Read the model definition and answer for the solid it produces. Units are mm, in the model's axes. A direction names the side the tool comes from. Coordinates: 2 decimals unless noted, no trailing zeros. Loops run counter-clockwise (first coordinate to the right, second up) from the corner with the lowest first, then second, coordinate; pieces in that order, holes last. Notation, with made-up numbers: (-20.75, 49) - (3.25, 49) arc R29 ccw to (3.25, 77) - close; hole circle Ø3 at (-30, -3). An arc over 180 degrees is marked (long way). One line per question, with ' | ' between items. Start each with the question number.
Autodesk Inventor part; units mm, degrees
ref_plane "YZ Plane" through (0, 0, 0) normal (1, 0, 0) x (0, 1, 0)
ref_plane "XZ Plane" through (0, 0, 0) normal (0, 1, 0) x (-1, 0, 0)
ref_plane "XY Plane" through (0, 0, 0) normal (0, 0, 1) x (1, 0, 0)
sketch "Sketch1" plane through (0, 0, 0) normal (0, 1, 0) x (-1, 0, 0)
  line L0 (0, 0) -> (57, 0)
  line L1 (57, 0) -> (57, -77)
  line L2 (57, -77) -> (0, -77)
  line L3 (0, -77) -> (0, 0)
  line L4 (53.5, -3.5) -> (3.5, -3.5) construction
  line L5 (3.5, -3.5) -> (3.5, -73.5) construction
  line L6 (3.5, -73.5) -> (53.5, -73.5) construction
  line L7 (53.5, -73.5) -> (53.5, -3.5) construction
  line L8 (52, -5) -> (5, -5)
  line L9 (5, -5) -> (5, -72)
  line L10 (5, -72) -> (52, -72)
  line L11 (52, -72) -> (52, -5)
  circle A0 centre (53.5, -3.5) radius 1.8
  circle A1 centre (53.5, -73.5) radius 1.8
  circle A2 centre (3.5, -3.5) radius 1.8
  circle A3 centre (3.5, -73.5) radius 1.8
  dimension "d0" = 57
  dimension "d1" = 77
  dimension "d2" = 50
  dimension "d3" = 70
  dimension "d4" = 3.5
  dimension "d5" = 3.5
  dimension "d6" = 67
  dimension "d7" = 47
  dimension "d8" = 1.5
  dimension "d9" = 1.5
  dimension "d10" = 3.6
  dimension "d11" = 3.6
  dimension "d12" = 3.6
  dimension "d13" = 3.6
extrude "Extrusion1" add sketch "Sketch1" along normal blind 5 contours L0 L1 L2 L3 | L11 L10 L9 L8
sketch "Sketch3" plane through (0, 5, 0) normal (0, 1, 0) x (1, 0, 0)
  line L0 (-52, 5) -> (-5, 5)
  line L1 (-5, 5) -> (-5, 72)
  line L2 (-5, 72) -> (-52, 72)
  line L3 (-52, 72) -> (-52, 5)
  line L4 (-57, 77) -> (-57, 0)
  line L5 (-57, 0) -> (0, 0)
  circle A0 centre (-53.5, 3.5) radius 1.8 construction
  circle A1 centre (-53.5, 3.5) radius 4.75
  circle A2 centre (-53.5, 73.5) radius 1.8 construction
  circle A3 centre (-53.5, 73.5) radius 4.75
  circle A4 centre (-3.5, 3.5) radius 1.8 construction
  circle A5 centre (-3.5, 3.5) radius 4.75
  circle A6 centre (-3.5, 73.5) radius 1.8 construction
  circle A7 centre (-3.5, 73.5) radius 4.75
  line L6 (-49.5, 7.5) -> (-7.5, 7.5)
  line L7 (-7.5, 7.5) -> (-7.5, 69.5)
  line L8 (-7.5, 69.5) -> (-49.5, 69.5)
  line L9 (-49.5, 69.5) -> (-49.5, 7.5)
  point P0 (-5, 68.9931)
  point P1 (-8.0069, 72)
  point P2 (-48.9931, 72)
  point P3 (-52, 68.9931)
  point P4 (-52, 8.0069)
  point P5 (-48.9931, 5)
  point P6 (-8.0069, 5)
  point P7 (-5, 8.0069)
  dimension "d30" = 47
  dimension "d31" = 67
  dimension "d32" = 5
  dimension "d33" = 5
  dimension "d34" = 9.5
  dimension "d35" = 9.5
  dimension "d36" = 9.5
  dimension "d37" = 9.5
  dimension "d38" = 42
  dimension "d39" = 62
  dimension "d40" = 2.5
  dimension "d41" = 2.5
extrude "Extrusion2" add sketch "Sketch3" along normal blind 25 contours A1 L3 A3 L2 A7 L1 A5 L0
sketch "Sketch4" plane through (-48.9931, 5, -5) normal (0, 0, 1) x (1, 0, 0)
  line L0 (4.4931, 23) -> (22.4931, 23)
  line L1 (22.4931, 23) -> (22.4931, 17)
  line L2 (22.4931, 17) -> (4.4931, 17)
  line L3 (4.4931, 17) -> (4.4931, 23)
  line L4 (43.9931, 0) -> (43.9931, 25)
  line L5 (-8.0069, 0) -> (48.9931, 0)
  point P0 (48.9931, -5)
  dimension "d44" = 18
  dimension "d45" = 6
  dimension "d46" = 21.5
  dimension "d47" = 17
extrude "Extrusion3" cut sketch "Sketch4" against normal blind 10
sketch "Sketch5" plane through (0, 30, 0) normal (0, 1, 0) x (1, 0, 0)
  line L0 (-5, 68.9931) -> (-5, 8.0069)
  line L1 (-5, 42) -> (2, 42)
  line L2 (2, 42) -> (2, 35)
  line L3 (2, 35) -> (-5, 35)
  line L4 (-5, 35) -> (-5, 42)
  line L5 (-8.0069, 72) -> (-48.9931, 72)
  line L6 (0, 77) -> (-57, 77) construction
  line L7 (-28.5, 77) -> (-28.5, 0) construction
  line L8 (-57, 0) -> (0, 0) construction
  line L9 (-5, 38.5) -> (2, 38.5) construction
  line L10 (-1.5, 42) -> (-1.5, 35) construction
  circle A0 centre (-1.5, 38.5) radius 1.8
  line L11 (-52, 42) -> (-59, 42)
  line L12 (-59, 42) -> (-59, 35)
  line L13 (-59, 35) -> (-52, 35)
  line L14 (-52, 35) -> (-52, 42)
  line L15 (-52, 38.5) -> (-59, 38.5) construction
  line L16 (-55.5, 42) -> (-55.5, 35) construction
  circle A1 centre (-55.5, 38.5) radius 1.8
  dimension "d50" = 7
  dimension "d51" = 7
  dimension "d52" = 30
  dimension "d53" = 3.6
extrude "Extrusion4" add sketch "Sketch5" against normal blind 7
sketch "Sketch6" plane through (-52, 5, -68.9931) normal (-1, 0, 0) x (0, 0, 1)
  line L0 (38.4931, 23) -> (48.4931, 23)
  line L1 (48.4931, 23) -> (48.4931, 5)
  line L2 (48.4931, 5) -> (38.4931, 5)
  line L3 (38.4931, 5) -> (38.4931, 23)
  line L4 (63.9931, 0) -> (63.9931, 25)
  line L5 (33.9931, 25) -> (60.9861, 25)
  line L6 (60.9861, 0) -> (0, 0)
  point P0 (68.9931, -5)
  dimension "d56" = 15.5
  dimension "d57" = 10
  dimension "d58" = 2
  dimension "d59" = 5
extrude "Extrusion5" cut sketch "Sketch6" against normal blind 25
sketch "Sketch8" plane through (0, 5, 0) normal (0, 1, 0) x (1, 0, 0)
  line L0 (-7.5, 7.5) -> (-7.5, 69.5)
  line L1 (-7.5, 7.5) -> (-17.5, 7.5)
  line L2 (-17.5, 7.5) -> (-17.5, 15.5)
  line L3 (-17.5, 15.5) -> (-7.5, 15.5)
  line L4 (-7.5, 15.5) -> (-7.5, 7.5)
  line L5 (-7.5, 69.5) -> (-7.5, 7.5)
  line L6 (-7.5, 69.5) -> (-17.5, 69.5)
  line L7 (-17.5, 69.5) -> (-17.5, 61.5)
  line L8 (-17.5, 61.5) -> (-7.5, 61.5)
  line L9 (-7.5, 61.5) -> (-7.5, 69.5)
  point P0 (0, 0)
  dimension "d64" = 10
  dimension "d65" = 8
  dimension "d68" = 10
  dimension "d69" = 8
extrude "Extrusion6" cut sketch "Sketch8" against normal blind 10
properties part number "ESPBox"
1) Given pin 1 Ø5.5 at (x, y) = (-57, 28) entering from -Z; pin 2 Ø2 at (x, z) = (-28.5, -59) entering from +Y; pin 3 Ø1 at (y, z) = (4, -68.5) entering from +X, each flat-ended and moving along its own axis, determine where each tip first touches the part or whether it passes through.
2) The part is cut by section D-D on z = -10.5. Write down the section's boundary in (x, y), and give its area (3 significant figures).
3) The mould has two halves that part along X. Classify faces 1 (the flat face through (-17.5, 3, -66)), 2 (the cylindrical face through (-50.16, 17.32, -6.88)), 3 (the flat face through (-51, 19, -20.5)): released by +X, released by -X, zero draft, split by the parting line, or undercut.
4) The part is cut by section A-A on x = -34. Write down the section's boundary in (y, z), and give its area (3 significant figures).
5) The part is cut by section B-B on z = -38.5. Write down the section's boundary in (x, y).
6) The part is cut by section C-C on y = 16.5. Write down the section's boundary in (x, z).
7) Which of the six approach directions +Z, -Z, +X, -X, +Y, -Y give full straight-line access (tool end or side, diameter ignored) to faces 4 (the flat face through (-35, 22, -6)), 5 (the flat face through (-1, 27, -35)), 6 (the flat face through (-57, 23, -40)), 7 (the cylindrical face through (-55.734, 26.549, -40.285))?
8) Find the intervals of material crossed by line 1 along Z through (x, y) = (-3.5, 3.3); line 2 along X through (y, z) = (2.5, -73.5); line 3 along X through (y, z) = (3.5, -69), in increasing order. Write a range as from..to.
Answer below:
1) pin 1: z = -42 | pin 2: y = 5 | pin 3: x = 0
2) outline: (-57, 0) - (-17.5, 0) - (-17.5, 5) - (-49.5, 5) - (-49.5, 30) - (-52, 30) - (-52, 5) - (-57, 5) - close; (-7.5, 0) - (0, 0) - (0, 5) - (-5, 5) - (-5, 30) - (-7.5, 30) - close | area: 360 mm2
3) face 1: undercut | face 2: released by -X | face 3: zero draft
4) outline: (0, -77) - (5, -77) - (5, -72) - (30, -72) - (30, -69.5) - (5, -69.5) - (5, -7.5) - (22, -7.5) - (22, -5) - (5, -5) - (5, 0) - (0, 0) - close; (28, -7.5) - (30, -7.5) - (30, -5) - (28, -5) - close | area: 495 mm2
5) outline: (-59, 23) - (-57.3, 23) - (-57.3, 30) - (-59, 30) - close; (-57, 0) - (0, 0) - (0, 5) - (-5, 5) - (-5, 23) - (-3.3, 23) - (-3.3, 30) - (-7.5, 30) - (-7.5, 5) - (-49.5, 5) - (-49.5, 30) - (-53.7, 30) - (-53.7, 23) - (-52, 23) - (-52, 5) - (-57, 5) - close; (0.3, 23) - (2, 23) - (2, 30) - (0.3, 30) - close
6) outline: (-52, -68.99) arc R4.75 cw to (-48.99, -72) - (-8.01, -72) arc R4.75 cw to (-5, -68.99) - (-5, -8.01) arc R4.75 cw to (-8.01, -5) - (-48.99, -5) arc R4.75 cw to (-52, -8.01) - (-52, -20.5) - (-49.5, -20.5) - (-49.5, -7.5) - (-7.5, -7.5) - (-7.5, -69.5) - (-49.5, -69.5) - (-49.5, -30.5) - (-52, -30.5) - close
7) face 4: +Z | face 5: +Z, +X, +Y | face 6: +Z, -Z, -X | face 7: +Y
8) line 1: -77..-75.3, -71.7..-5.3, -1.7..0 | line 2: -57..-55.3, -51.7..-5.3, -1.7..0 | line 3: -57..-17.5, -7.5..0
